Design review of the part built by this model. Coordinates are the model's own, in mm. Face numbers are marked on the shaded views. A direction names the side the tool comes from. Round coordinates to 2 decimals unless told otherwise and drop trailing zeros. Order: outer loops, then holes, each group sorted by start corner. A loop starts at its lowest first (then second) coordinate and runs counter-clockwise, first axis right, second up.
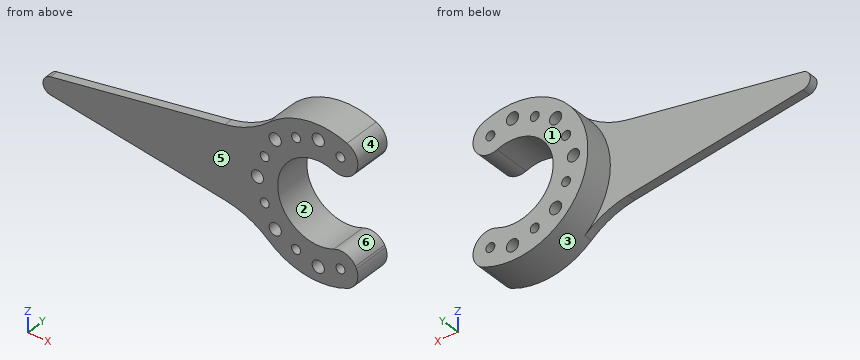
from build123d import *

# Parameters (mm, degrees)
SKETCH4_R           = 26
SKETCH4_R_2         = 2.1
SKETCH4_R_3         = 1.55
BOSS_EXTRUDE1_DEPTH = 13
SKETCH5_OUTSIDE_W   = 68.936
SKETCH5_OUTSIDE_H   = 68.936
CUT_EXTRUDE1_DEPTH  = 40
BOSS_EXTRUDE2_START = -3
BOSS_EXTRUDE2_DEPTH = 3


with BuildPart() as part:
    # Sketch4 → Boss-Extrude1 (new body)
    with BuildSketch(Plane(origin=(0, 0, 3), x_dir=(1, 0, 0), z_dir=(0, -1, 0))):
        with Locations(Location((0, -3, 0), (0, 0, 90))):
            Circle(SKETCH4_R)
        with Locations(Location((0, 18, 0), (0, 0, 90))):
            Circle(SKETCH4_R_2, mode=Mode.SUBTRACT)
        with Locations(Location((7.653668647, 15.47759065, 0), (0, 0, 90))):
            Circle(SKETCH4_R_3, mode=Mode.SUBTRACT)
        with Locations(Location((14.849242405, 11.849242405, 0), (0, 0, 90))):
            Circle(SKETCH4_R_2, mode=Mode.SUBTRACT)
        with Locations(Location((18.47759065, 4.653668647, 0), (0, 0, 90))):
            Circle(SKETCH4_R_3, mode=Mode.SUBTRACT)
        with Locations(Location((21, -3, 0), (0, 0, 90))):
            Circle(SKETCH4_R_2, mode=Mode.SUBTRACT)
        with Locations(Location((18.47759065, -10.653668647, 0), (0, 0, 90))):
            Circle(SKETCH4_R_3, mode=Mode.SUBTRACT)
        with Locations(Location((14.849242405, -17.849242405, 0), (0, 0, 90))):
            Circle(SKETCH4_R_2, mode=Mode.SUBTRACT)
        with Locations(Location((7.653668647, -21.47759065, 0), (0, 0, 90))):
            Circle(SKETCH4_R_3, mode=Mode.SUBTRACT)
        with Locations(Location((0, -24, 0), (0, 0, 90))):
            Circle(SKETCH4_R_2, mode=Mode.SUBTRACT)
        with Locations(Location((-7.653668647, -21.47759065, 0), (0, 0, 90))):
            Circle(SKETCH4_R_3, mode=Mode.SUBTRACT)
        with Locations(Location((-14.849242405, -17.849242405, 0), (0, 0, 90))):
            Circle(SKETCH4_R_2, mode=Mode.SUBTRACT)
        with Locations(Location((-18.47759065, -10.653668647, 0), (0, 0, 90))):
            Circle(SKETCH4_R_3, mode=Mode.SUBTRACT)
        with Locations(Location((-21, -3, 0), (0, 0, 90))):
            Circle(SKETCH4_R_2, mode=Mode.SUBTRACT)
        with Locations(Location((-18.47759065, 4.653668647, 0), (0, 0, 90))):
            Circle(SKETCH4_R_3, mode=Mode.SUBTRACT)
        with Locations(Location((-14.849242405, 11.849242405, 0), (0, 0, 90))):
            Circle(SKETCH4_R_2, mode=Mode.SUBTRACT)
        with Locations(Location((-7.653668647, 15.47759065, 0), (0, 0, 90))):
            Circle(SKETCH4_R_3, mode=Mode.SUBTRACT)
    extrude(amount=BOSS_EXTRUDE1_DEPTH)

    # Sketch5 outside → Cut-Extrude1 (cut, through all)
    with BuildSketch(Plane.XZ.offset(13)):
        Rectangle(SKETCH5_OUTSIDE_W, SKETCH5_OUTSIDE_H)
        with BuildLine():
            ThreePointArc((5.357568053, 12.934313455), (-14, 0), (5.357568053, -12.934313455))
            ThreePointArc((5.357568053, -12.934313455), (13.196945842, -16.181490056), (9.949769241, -24.020867845))
            ThreePointArc((9.949769241, -24.020867845), (-26, 0), (9.949769241, 24.020867845))
            ThreePointArc((9.949769241, 24.020867845), (13.196945842, 16.181490056), (5.357568053, 12.934313455))
        make_face(mode=Mode.SUBTRACT)
    extrude(amount=-CUT_EXTRUDE1_DEPTH, mode=Mode.SUBTRACT)

    # Sketch6 → Boss-Extrude2 (add)
    with BuildSketch(Plane.XZ.offset(13).offset(BOSS_EXTRUDE2_START)):
        with BuildLine():
            Line((-92.43614906, 3), (-32.213868088, 12.5))
            ThreePointArc((-32.213868088, 12.5), (-24.170350504, 14.962836151), (-17.126817214, 19.562007364))
            ThreePointArc((-17.126817214, 19.562007364), (-26, 0), (-17.126817214, -19.562007364))
            ThreePointArc((-17.126817214, -19.562007364), (-24.170350504, -14.962836151), (-32.213868088, -12.5))
            Line((-32.213868088, -12.5), (-92.43614906, -3))
            ThreePointArc((-92.43614906, -3), (-95, 0), (-92.43614906, 3))
        make_face()
    extrude(amount=BOSS_EXTRUDE2_DEPTH)


solid = part.part
1) Take a section at B-B on x = 0. Give the boundary of the cut face in (y, z), plus the area to 3 significant figures.
Results:
outline: (-13, -26) - (0, -26) - (0, -23.1) - (-13, -23.1) - close; (-13, -18.9) - (0, -18.9) - (0, -14) - (-13, -14) - close; (-13, 14) - (0, 14) - (0, 18.9) - (-13, 18.9) - close; (-13, 23.1) - (0, 23.1) - (0, 26) - (-13, 26) - close
area: 203 mm2
2) For the marked faces 5 and 6, list the 3-axis set-ups (+Z, -Z, +X, -X, +Y, -Y) from which the entire face can be reached by the end or side of a thin tool; tool diameter is ignored.
Results:
face 5: +Z, -Z, +X, -X, -Y
face 6: +Y, -Y
3) Take a section at D-D on y = -8.75. State how many separate pieces and enclosed holes the cut face has, plus the area to 3 significant figures.
Results:
separate pieces: 1
enclosed holes: 11
area: 941 mm2
4) Take a section at A-A on z = 0. Give the boundary of the cut face in (x, y).
Results:
outline: (-95, -13) - (-23.1, -13) - (-23.1, 0) - (-26, 0) - (-26, -10) - (-95, -10) - close; (-18.9, -13) - (-14, -13) - (-14, 0) - (-18.9, 0) - close
5) Take a section at C-C on x = -21. Give the boundary of the cut face in (y, z), plus the area to 3 significant figures.
Results:
outline: (-13, -16.69) - (-10, -16.69) - (-10, -15.33) - (0, -15.33) - (0, -2.1) - (-13, -2.1) - close; (-13, 2.1) - (0, 2.1) - (0, 15.33) - (-10, 15.33) - (-10, 16.69) - (-13, 16.69) - close
area: 352 mm2
6) The part is to be moulded in two halves that separate along X. For the marked faces 1, 2, 3 and 4, say which applies: released by +X, released by -X, zero draft, split by the parting line, or undercut.
Results:
face 1: zero draft
face 2: undercut
face 3: split by the parting line
face 4: released by +X
7) Clearance check with flat-ended pins moving along their axes: P1, Ø2.5, axis at x = 7.65, z = -18.48, coming from the +Y side; P2, Ø2, axis at x = -50.5, z = 6.5, coming from the +Y side; P3, Ø1.5, axis at x = -44.5, y = -11.5, coming from the -Z side. State where each tip first meets the part, or that it passes through.
Results:
P1: passes through
P2: stops at y = -10
P3: stops at z = -10.68
8) To check wall thickness, follow line 1 along Z through (x, y) = (-7.5, -12.5); line 2 along X through (y, z) = (-0.5, 0); line 3 along X through (y, z) = (-0.75, 18). State the ranges of each line that lie inside material, in increasing order.
Results:
line 1: z = -24.89 to -20.02, -16.94 to -11.82, 11.82 to 16.94, 20.02 to 24.89
line 2: x = -26 to -23.1, -18.9 to -14
line 3: x = -18.76 to -9.13, -6.18 to 6.18, 9.13 to 13.63
